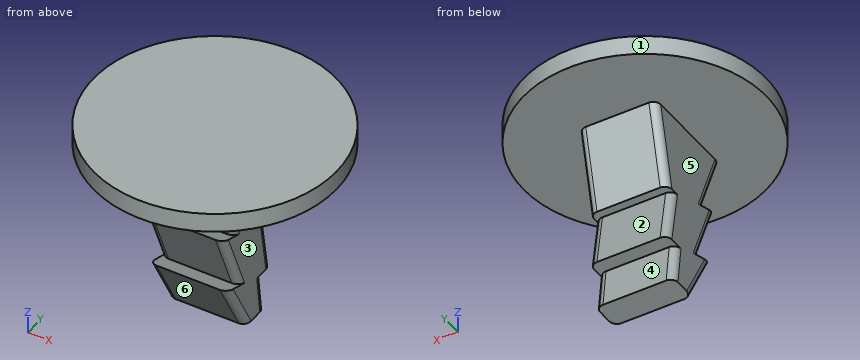
```python
from build123d import *

# Parameters (mm, degrees)
F0_R          = 12.5
F1_DEPTH      = 2
F3_DEPTH      = 4
F3_DEPTH_BACK = 4
F4_R          = 0.75


with BuildPart() as f1:
    # F0 (on Top) → F1 (new body)
    with BuildSketch(Plane.XY):
        Circle(F0_R)
    extrude(amount=F1_DEPTH)

    # F2 (on Right) → F3 (join, two sides)
    with BuildSketch(Plane.YZ) as f3_sk:
        Polygon((4.633974, 0), (-6, 0), (-3.322237, -6.605754), (-5.188579, -6.005191), (-2.479827, -12.687395), (-4.499659, -12.065352), (-1.3, -18), (0, -18), (1.75, -18), (1.246213, -13.898331), (2.769501, -13.898331), (1.839659, -8.247796), (2.752447, -8.247796), align=None)
    extrude(amount=F3_DEPTH)
    extrude(f3_sk.sketch, amount=-F3_DEPTH_BACK)

    # F4
    f4_edges = [f1.edges().sort_by_distance(p)[0] for p in [
        (-4, 3.693211, -4.123898),
        (-4, -4.661119, -3.302877),
        (-4, 2.30458, -11.073063),
        (-4, -3.834203, -9.346293),
        (-4, 1.498106, -15.949165),
        (-4, -2.899829, -15.032676),
        (4, 3.693211, -4.123898),
        (4, 2.30458, -11.073063),
        (4, -2.899829, -15.032676),
        (4, 1.498106, -15.949165),
        (4, -3.834203, -9.346293),
        (4, -4.661119, -3.302877),
    ]]
    fillet(f4_edges, radius=F4_R)


solid = f1.part
```
Work out the finished part from the listing and answer in its coordinate system (mm). Face numbers are marked on the shaded views. A direction names the side the tool comes from. Round coordinates to 2 decimals unless told otherwise and drop trailing zeros. Order: outer loops, then holes, each group sorted by start corner. A loop starts at its lowest first (then second) coordinate and runs counter-clockwise, first axis right, second up.
Q1. A cutting plane is placed at B-B, the plane y = 0. Determine the outline of the cut face in (x, z).
Solution:
outline: (-12.5, 0) - (-4, 0) - (-4, -18) - (4, -18) - (4, 0) - (12.5, 0) - (12.5, 2) - (-12.5, 2) - close
Q2. A tool of negligible diameter and unlimited length cuts with its end or side. For the marked faces 1, 2 and 3, from which of +Z, -Z, +X, -X, +Y, -Y can it reach the whole face along a straight path? Write none if from no direction.
Solution:
face 1: +Z, -Z
face 2: +X, -X, +Y
face 3: -Z, +X, +Y, -Y
Q3. Find the intervals of material crossed by line 1 along Z through (x, y) = (1.5, 11.75); line 2 along X through (y, z) = (-1.5, -3); line 3 along Y through (x, z) = (3.5, -3.25), in increasing order.
Solution:
line 1: z = 0 to 2
line 2: x = -4 to 4
line 3: y = -4.64 to 3.85
Q4. The mould has two halves that part along Z. Classify the marked faces 4, 5 and 6: pulls with the +Z half, pulls with the -Z half, needs draft (parallel to the pull), parting line crosses it, or undercut.
Solution:
face 4: undercut
face 5: needs draft
face 6: pulls with the -Z half
Q5. A cutting plane is placed at C-C, the plane y = -7.5. Determine the outline of the cut face in (x, z), then the cut area to 3 significant figures.
Solution:
outline: (-10, 0) - (10, 0) - (10, 2) - (-10, 2) - close
area: 40.0 mm2
Q6. A cutting plane is placed at A-A, the plane x = 0. Determine the outline of the cut face in (y, z).
Solution:
outline: (-12.5, 0) - (-6, 0) - (-3.32, -6.61) - (-5.19, -6.01) - (-2.48, -12.69) - (-4.5, -12.07) - (-1.3, -18) - (1.75, -18) - (1.25, -13.9) - (2.77, -13.9) - (1.84, -8.25) - (2.75, -8.25) - (4.63, 0) - (12.5, 0) - (12.5, 2) - (-12.5, 2) - close
Q7. A cutting plane is placed at D-D, the plane x = 10.5. Determine the outline of the cut face in (y, z), then the cut area to 3 significant figures.
Solution:
outline: (-6.78, 0) - (6.78, 0) - (6.78, 2) - (-6.78, 2) - close
area: 27.1 mm2
Q8. Given pin 1 Ø1 at (y, z) = (4, -7) entering from -X; pin 2 Ø8 at (x, z) = (1.5, -12.5) entering from +Y; pin 3 Ø5 at (x, y) = (9, -8.5) entering from -Z; pin 4 Ø7 at (y, z) = (0, -11.5) entering from -X, each flat-ended and moving along its own axis, determine where each tip first touches the part or whether it passes through.
Solution:
pin 1: passes through
pin 2: stops at y = 2.77
pin 3: stops at z = 0
pin 4: stops at x = -4
